Can you work these out from the model? Positions are in its coordinate system, mm. A direction names the side the tool comes from. Give positions to 0.01 mm unless a question says otherwise; leave off trailing zeros. Loops run counter-clockwise (first coordinate to the right, second up) from the corner with the lowest first, then second, coordinate; pieces in that order, holes last. Notation, with made-up numbers: (44, 78) - (89, 78) arc R16 ccw to (89, 83) - close; hole circle Ø5 at (72.25, 37). An arc over 180 degrees is marked (long way). Answer in a Markdown table with one row per item.
Autodesk Fusion 360 part; units mm, degrees
sketch "Szkic1" plane through (0, 0, 0) normal (0, 0, 1) x (1, 0, 0)
  line L0 (0, 0) -> (158.35, 0)
  line L1 (158.35, 0) -> (158.35, 93)
  line L2 (158.35, 93) -> (0, 93)
  line L3 (0, 93) -> (0, 0)
  line L4 (3, 5) -> (3, 3)
  line L5 (3, 3) -> (5, 3)
  line L6 (3, 3) -> (155.35, 3)
  line L7 (155.35, 3) -> (155.35, 90)
  line L8 (155.35, 90) -> (3, 90)
  line L9 (3, 90) -> (3, 3)
  dimension "d1" = 158.35
  dimension "d2" = 93
  dimension "d3" = 152.35
  dimension "d4" = 87
extrude "Wyciągnięcie proste1" add sketch "Szkic1" along normal blind 150
sketch "Szkic2" plane through (0, 90, 0) normal (0, -1, 0) x (1, 0, 0)
  line L0 (3, 0) -> (155.35, 0)
  line L1 (155.35, 0) -> (155.35, 150)
  line L2 (155.35, 150) -> (3, 150)
  line L3 (3, 150) -> (3, 0)
  line L4 (79.175, 150) -> (77.175, 150)
  line L5 (77.175, 150) -> (81.175, 150)
  line L6 (81.175, 150) -> (81.175, 0)
  line L7 (81.175, 0) -> (77.175, 0)
  line L8 (77.175, 0) -> (77.175, 150)
  dimension "d7" = 2
  dimension "d8" = 4
extrude "Wyciągnięcie proste2" add sketch "Szkic2" along normal blind 87 contours L0 L2 L4 L5 L6 L7 L8
sketch "Szkic3" plane through (0, 0, 0) normal (0, -1, 0) x (1, 0, 0)
  line L0 (0, 0) -> (158.35, 0)
  line L1 (158.35, 0) -> (158.35, 150)
  line L2 (158.35, 150) -> (0, 150)
  line L3 (0, 150) -> (0, 0)
sketch "Szkic4" plane through (0, 0, 0) normal (0, 0, -1) x (1, 0, 0)
  line L0 (81.175, -3) -> (155.35, -3)
  line L1 (155.35, -3) -> (155.35, -90)
  line L2 (155.35, -90) -> (81.175, -90)
  line L3 (81.175, -90) -> (81.175, -3)
  line L4 (77.175, -3) -> (77.175, -90)
  line L5 (77.175, -90) -> (3, -90)
  line L6 (3, -90) -> (3, -3)
  line L7 (3, -3) -> (77.175, -3)
  line L8 (0, 0) -> (0, -93)
  line L9 (0, -93) -> (158.35, -93)
  line L10 (158.35, -93) -> (158.35, 0)
  line L11 (158.35, 0) -> (0, 0)
  line L12 (0, 0) -> (158.35, 0)
  line L13 (158.35, 0) -> (158.35, -93)
  line L14 (158.35, -93) -> (0, -93)
  line L15 (0, -93) -> (0, 0)
extrude "Wyciągnięcie proste3" add sketch "Szkic4" against normal blind 3 contours L0 L1 L2 L3 | L4 L5 L6 L7
sketch "Szkic5" plane through (0, 0, 0) normal (0, -1, 0) x (1, 0, 0)
  line L0 (40, 15) -> (38.0507, 15)
  line L1 (38.0507, 15) -> (28.0507, 15)
  line L2 (28.0507, 15) -> (48.0507, 15)
  line L3 (48.0507, 15) -> (48.0507, 135)
  line L4 (48.0507, 135) -> (28.0507, 135)
  line L5 (28.0507, 135) -> (28.0507, 15)
  line L6 (131.9493, 135) -> (131.9493, 15)
  line L7 (120, 15) -> (121.9493, 15)
  line L8 (111.9493, 135) -> (131.9493, 135)
  line L9 (121.9493, 15) -> (131.9493, 15)
  line L10 (131.9493, 15) -> (111.9493, 15)
  line L11 (111.9493, 15) -> (111.9493, 135)
  dimension "d13" = 10
  dimension "d14" = 20
  dimension "d15" = 120
extrude "Wyciągnięcie proste4" cut sketch "Szkic5" against normal blind 10
sketch "Szkic6" plane through (0, 0, 3) normal (0, 0, 1) x (-1, 0, 0)
  line L0 (-3, -90) -> (-3, -3)
  line L1 (-3, -3) -> (-77.175, -3)
  line L2 (-77.175, -3) -> (-77.175, -90)
  line L3 (-77.175, -90) -> (-3, -90)
  line L4 (-77.175, -3) -> (-77.175, -90)
  line L5 (-77.175, -90) -> (-3, -90)
  line L6 (-3, -90) -> (-3, -3)
  line L7 (-3, -90) -> (-5, -90)
sketch "Szkic7" plane through (0, 0, 3) normal (0, 0, 1) x (-1, 0, 0)
  line L0 (-77.175, -90) -> (-77.175, -3)
  line L1 (-77.175, -3) -> (-77.175, -5)
  line L2 (-75.175, -5) -> (-5, -5)
  line L3 (-5, -5) -> (-5, -88)
  line L4 (-5, -88) -> (-75.175, -88)
  line L5 (-75.175, -88) -> (-75.175, -5)
  point P0 (-5, -90)
  point P1 (-77.175, -3)
  dimension "d18" = 2
extrude "Wyciągnięcie proste5" cut sketch "Szkic7" against normal blind 10
Q1. Imagine slicing it at B-B, the plane y = 13. Write out the boundary of the cut face in (x, z) (3 decimals), and give its area (3 significant figures).
Checked values:
| item | result |
|---|---|
| outline | (0, 0) - (5, 0) - (5, 3) - (3, 3) - (3, 150) - (0, 150) - close; (75.175, 0) - (158.35, 0) - (158.35, 150) - (155.35, 150) - (155.35, 3) - (81.175, 3) - (81.175, 150) - (77.175, 150) - (77.175, 3) - (75.175, 3) - close |
| area | 1,730 mm² |
Q2. On a 3-axis mill with a long thin cutter (end or side, diameter ignored), from which of +Z, -Z, +X, -X, +Y, -Y can I reach the whole of each face in a straight line? I mean faces 1 (the face through (78, 0, 74)), 2 (the face through (4, 46, 3)). Say none if no direction works.
Checked values:
| item | result |
|---|---|
| face 1 | +Z, -Z, +X, -X, -Y |
| face 2 | +Z |
Q3. If we mould it in two halves opening along X, with no side actions, what happens to faces 3 (the face through (119, 90, 75)), 4 (the face through (0, 47, 74)), 5 (the face through (80, 93, 74)), 6 (the face through (3, 47, 75))? For each: released by +X, released by -X, zero draft, split by the parting line, or undercut.
Checked values:
| item | result |
|---|---|
| face 3 | undercut |
| face 4 | released by -X |
| face 5 | zero draft |
| face 6 | undercut |
Q4. For pin 1 (12 mm diameter, centred on x = 35, z = 122.5, fed in from -Y); pin 2 (1 mm diameter, centred on x = 82.5, y = 34, fed in from +Z), each with a flat end and sliding along its axis, tell me the tip position at first contact or that it passes through.
Checked values:
| item | result |
|---|---|
| pin 1 | stops at y = 90 |
| pin 2 | stops at z = 3 |
Q5. Imagine slicing it at A-A, the plane x = 62. Write out the boundary of the cut face in (y, z), and give its area (3 significant figures).
Checked values:
| item | result |
|---|---|
| outline | (0, 0) - (5, 0) - (5, 3) - (3, 3) - (3, 150) - (0, 150) - close; (88, 0) - (93, 0) - (93, 150) - (90, 150) - (90, 3) - (88, 3) - close |
| area | 912 mm² |
Q6. Imagine slicing it at C-C, the plane x = 98.5. Write out the boundary of the cut face in (y, z).
Checked values:
| item | result |
|---|---|
| outline | (0, 0) - (93, 0) - (93, 150) - (90, 150) - (90, 3) - (3, 3) - (3, 150) - (0, 150) - close |
Q7. If I drill on line 1 (X direction, y = 33, z = 35) (3 decimals); line 2 (Y direction, x = 18.5, z = 73.5); line 3 (Y direction, x = 120, z = 122), over which ranges is the centre line in solid material (lowest first)? Write a range as [from, to].
Checked values:
| item | result |
|---|---|
| line 1 | x = [0, 3], [77.175, 81.175], [155.35, 158.35] |
| line 2 | y = [0, 3], [90, 93] |
| line 3 | y = [90, 93] |
Q8. Imagine slicing it at D-D, the plane z = 105.5. Write out the boundary of the cut face in (x, y) (3 decimals).
Checked values:
| item | result |
|---|---|
| outline | (0, 0) - (28.051, 0) - (28.051, 3) - (3, 3) - (3, 90) - (77.175, 90) - (77.175, 3) - (48.051, 3) - (48.051, 0) - (111.949, 0) - (111.949, 3) - (81.175, 3) - (81.175, 90) - (155.35, 90) - (155.35, 3) - (131.949, 3) - (131.949, 0) - (158.35, 0) - (158.35, 93) - (0, 93) - close |
